```python
from build123d import *

# Parameters (mm, degrees)
SKETCH1_W               = 13
SKETCH1_H               = 8
BOSS_EXTRUDE1_DEPTH     = 3
CUT_EXTRUDE1_DEPTH      = 16.556349186
CUT_EXTRUDE1_DEPTH_BACK = 16.556349186
CUT_EXTRUDE2_DEPTH      = 16.556349186
CUT_EXTRUDE2_DEPTH_BACK = 16.556349186
SKETCH4_R               = 1.8
CUT_EXTRUDE3_DEPTH      = 0.8
SKETCH5_W               = 8
SKETCH5_H               = 1.1
BOSS_EXTRUDE2_DEPTH     = 2
FILLET1_R               = 4
SKETCH6_W               = 0.576923077
SKETCH6_H               = 3
CUT_EXTRUDE4_DEPTH      = 0.4


with BuildPart() as part:
    # Sketch1 → Boss-Extrude1 (new body)
    with BuildSketch(Plane(origin=(0, 0, 0), x_dir=(1, 0, 0), z_dir=(0, 1, 0))):
        with Locations((6.5, 4)):
            Rectangle(SKETCH1_W, SKETCH1_H)
    extrude(amount=BOSS_EXTRUDE1_DEPTH)

    # Sketch2 → Cut-Extrude1 (cut, two sides: drawn at the far end of the back side and taken through both)
    with BuildSketch(Plane.XY.offset(-CUT_EXTRUDE1_DEPTH_BACK)):
        Polygon((0, 0), (0.6, 3), (0, 3), align=None)
        Polygon((13, 0), (12.4, 3), (13, 3), align=None)
    extrude(amount=CUT_EXTRUDE1_DEPTH + CUT_EXTRUDE1_DEPTH_BACK, mode=Mode.SUBTRACT)

    # Sketch3 → Cut-Extrude2 (cut, two sides: drawn at the far end of the back side and taken through both)
    with BuildSketch(Plane(origin=(0, 0, 0), x_dir=(0, 0, -1), z_dir=(1, 0, 0)).offset(-CUT_EXTRUDE2_DEPTH_BACK)):
        Polygon((0, 0), (0.6, 3), (0, 3), align=None)
        Polygon((8, 3), (7.4, 3), (8, 0), align=None)
    extrude(amount=CUT_EXTRUDE2_DEPTH + CUT_EXTRUDE2_DEPTH_BACK, mode=Mode.SUBTRACT)

    # Sketch4 → Cut-Extrude3 (cut)
    with BuildSketch(Plane.XZ):
        with Locations(Location((6.50000125, -3.75, 0), (0, 0, 270))):
            Circle(SKETCH4_R)
    extrude(amount=-CUT_EXTRUDE3_DEPTH, mode=Mode.SUBTRACT)

    # Sketch5 → Boss-Extrude2 (add)
    with BuildSketch(Plane.XZ):
        with Locations((6.500011, -7.45)):
            Rectangle(SKETCH5_W, SKETCH5_H)
    extrude(amount=BOSS_EXTRUDE2_DEPTH)

    # Fillet1
    # the kernel refuses this fillet: 4 mm, written as the material it takes off along each edge
    with BuildSketch(Plane(origin=(10.500011, -2, -16.660254038), x_dir=(0, 1, 0), z_dir=(0, 0, 1)), Plane(origin=(2.500011, -2, 1.760254038), x_dir=(0, 1, 0), z_dir=(0, 0, -1))) as fillet1_piece_1:
        with BuildLine():
            CenterArc((4, 3.464101615), FILLET1_R, 180, 60)
            Line((0, 3.464101615), (-0.08, 3.464101615))
            Line((-0.08, 3.464101615), (-0.08, 0))
            Line((-0.08, 0), (0, -0.08))
            ThreePointArc((0, -0.08), (1, -0.08), (1.96, -0.069282032))
            Line((1.96, -0.069282032), (2, 0))
        make_face()
    extrude(amount=18.420508076, mode=Mode.SUBTRACT)

    # Sketch6 → Cut-Extrude4 (cut)
    with BuildSketch(Plane(origin=(0, 3, 0), x_dir=(1, 0, 0), z_dir=(0, 1, 0))):
        Polygon((3.219165588, 2.557267472), (2.50101655, 5.557267472), (3.092362704, 5.557267472), (3.558708858, 3.496570357), (4.052098281, 5.557267472), (4.839357896, 5.557267472), (5.327939627, 3.461714587), (5.793083858, 5.557267472), (6.385631934, 5.557267472), (5.68070405, 2.557267472), (4.966160781, 2.557267472), (4.443324242, 4.800055934), (3.906665588, 2.557267472), align=None)
        with Locations((6.981785781, 4.057267472)):
            Rectangle(SKETCH6_W, SKETCH6_H)
        Polygon((7.885631934, 2.557267472), (7.885631934, 5.557267472), (8.488396358, 5.557267472), (9.693324242, 3.584911703), (9.693324242, 5.557267472), (10.270247319, 5.557267472), (10.270247319, 2.557267472), (9.648853088, 2.557267472), (8.462555011, 4.498373241), (8.462555011, 2.557267472), align=None)
    extrude(amount=-CUT_EXTRUDE4_DEPTH, mode=Mode.SUBTRACT)


solid = part.part
```
Part model, mm, in its own coordinate system. A direction names the side the tool comes from. Round coordinates to 2 decimals unless told otherwise and drop trailing zeros. Order: outer loops, then holes, each group sorted by start corner. A loop starts at its lowest first (then second) coordinate and runs counter-clockwise, first axis right, second up. Notation, with made-up numbers: M 25.25,-13 L 66.25,-13 A20 ccw 66.25,-6 Z; hole C 78,16.5 d6. An arc over 180 degrees is marked long. Put each result on its own line as item: value. Start each with the question number.
1. Drill centre lines: probe 1 along Y at (x, z) = (3.5, -4.75); probe 2 along Y at (x, z) = (8.25, -5.5); probe 3 along X at (y, z) = (0.45, -3.75). Where is each one in solid material? Low to high. Write a range as [from, to].
2. Slice it at B-B on z = -2.25. List the corners of the cut face in (x, y), then the cut area to 3 significant figures.
3. Drop a flat-ended pin along its axis: pin 1 (3 mm diameter, centred on x = 10, z = -4.5, fed in from -Y). Give the stop position or say it passes through.
4. Slice it at A-A on y = 1.7. List the corners of the cut face in (x, z), then the cut area to 3 significant figures.
5. Tool access for faces 1 (the face through (6.5, -2, -7.4)), 2 (the face through (3.99, -1.48, -7.44)), 3 (the face through (4, 2.6, -4)), 4 (the face through (5.811, 0.394, -5.413)), 5 (the face through (6, -1, -6.9)): list every direction of +Z, -Z, +X, -X, +Y, -Y with a clear straight run to the whole face (end or side of a thin tool).
6. Slice it at C-C on z = -6.75. List the corners of the cut face in (x, y).
7. Two-plate mould, pull along Z, no slides. Class faces 6 (the face through (9.01, -1.48, -7.46)), 7 (the face through (6, -1, -8)), 8 (the face through (7, 0.8, -4)): +Z half, -Z half, draft (parallel to the pull), parting line (faces both ways), or undercut.
Findings:
1. probe 1: [0, 3]
1. probe 2: [0, 2.6]
1. probe 3: [0.09, 4.7], [8.3, 12.91]
2. outline: M 0,0 L 5.51,0 L 5.51,0.8 L 7.49,0.8 L 7.49,0 L 13,0 L 12.4,3 L 0.6,3 Z
2. area: 35.6 mm2
3. pin 1: y = 0
4. outline: M 0.34,-7.66 L 12.66,-7.66 L 12.66,-0.34 L 0.34,-0.34 Z
4. area: 90.2 mm2
5. face 1: +Z, -Z, +X, -X, -Y
5. face 2: +Z, -Z, -X, -Y
5. face 3: +Y
5. face 4: -Y
5. face 5: +Z, +X, -X, -Y
6. outline: M 0,0 L 13,0 L 12.4,3 L 0.6,3 Z
7. face 6: draft
7. face 7: -Z half
7. face 8: undercut
